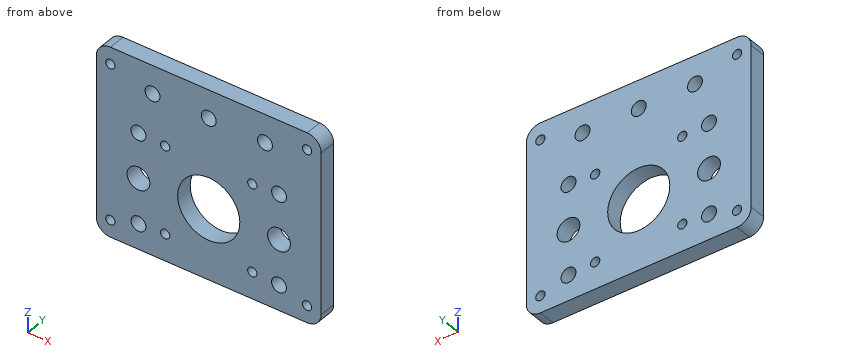
from build123d import *

# Parameters (mm, degrees)
SKETCH_1_R      = 11.05
SKETCH_1_R_2    = 1.65
SKETCH_1_R_3    = 4.05
SKETCH_1_R_4    = 2.65
EXTRUDE_1_DEPTH = 6


with BuildPart() as part:
    # 草图1 → 凸台-拉伸1 (new body)
    with BuildSketch(Plane(origin=(0, 0, 0), x_dir=(1, 0, 0), z_dir=(0, 1, 0))):
        with BuildLine():
            Line((-35, -42), (35, -42))
            ThreePointArc((35, -42), (38.535533906, -40.535533906), (40, -37))
            Line((40, -37), (40, 20))
            ThreePointArc((40, 20), (38.535533906, 23.535533906), (35, 25))
            Line((35, 25), (-35, 25))
            ThreePointArc((-35, 25), (-38.535533906, 23.535533906), (-40, 20))
            Line((-40, 20), (-40, -37))
            ThreePointArc((-40, -37), (-38.535533906, -40.535533906), (-35, -42))
        make_face()
        with Locations(Location((0, 0, 0), (0, 0, 270))):
            Circle(SKETCH_1_R, mode=Mode.SUBTRACT)
        with Locations(Location((-15.5, 15.5, 0), (0, 0, 270))):
            Circle(SKETCH_1_R_2, mode=Mode.SUBTRACT)
        with Locations(Location((15.5, 15.5, 0), (0, 0, 270))):
            Circle(SKETCH_1_R_2, mode=Mode.SUBTRACT)
        with Locations(Location((15.5, -15.5, 0), (0, 0, 270))):
            Circle(SKETCH_1_R_2, mode=Mode.SUBTRACT)
        with Locations(Location((-15.5, -15.5, 0), (0, 0, 270))):
            Circle(SKETCH_1_R_2, mode=Mode.SUBTRACT)
        with Locations(Location((-25, 0, 0), (0, 0, 270))):
            Circle(SKETCH_1_R_3, mode=Mode.SUBTRACT)
        with Locations(Location((-25, 16, 0), (0, 0, 270))):
            Circle(SKETCH_1_R_4, mode=Mode.SUBTRACT)
        with Locations(Location((-25, -16, 0), (0, 0, 90))):
            Circle(SKETCH_1_R_4, mode=Mode.SUBTRACT)
        with Locations(Location((25, 0, 0), (0, 0, 90))):
            Circle(SKETCH_1_R_3, mode=Mode.SUBTRACT)
        with Locations(Location((25, -16, 0), (0, 0, 270))):
            Circle(SKETCH_1_R_4, mode=Mode.SUBTRACT)
        with Locations(Location((25, 16, 0), (0, 0, 90))):
            Circle(SKETCH_1_R_4, mode=Mode.SUBTRACT)
        with Locations(Location((-20, -32, 0), (0, 0, 270))):
            Circle(SKETCH_1_R_4, mode=Mode.SUBTRACT)
        with Locations(Location((0, -32, 0), (0, 0, 270))):
            Circle(SKETCH_1_R_4, mode=Mode.SUBTRACT)
        with Locations(Location((20, -32, 0), (0, 0, 270))):
            Circle(SKETCH_1_R_4, mode=Mode.SUBTRACT)
        with Locations(Location((-35, 19, 0), (0, 0, 270))):
            Circle(SKETCH_1_R_2, mode=Mode.SUBTRACT)
        with Locations(Location((-35, -36, 0), (0, 0, 270))):
            Circle(SKETCH_1_R_2, mode=Mode.SUBTRACT)
        with Locations(Location((35, -36, 0), (0, 0, 90))):
            Circle(SKETCH_1_R_2, mode=Mode.SUBTRACT)
        with Locations(Location((35, 19, 0), (0, 0, 90))):
            Circle(SKETCH_1_R_2, mode=Mode.SUBTRACT)
    extrude(amount=EXTRUDE_1_DEPTH)


solid = part.part
The model under review builds one solid part; all positions refer to its coordinate system, in mm. Give positions to 0.01 mm unless a question says otherwise; leave off trailing zeros. Loops run counter-clockwise (first coordinate to the right, second up) from the corner with the lowest first, then second, coordinate; pieces in that order, holes last. Notation, with made-up numbers: (40, 42) -> (75, 42) arc R10 cw to (75, 59) -> close; hole circle Ø1 at (34.25, -29). An arc over 180 degrees is marked (long way). Answer as a JSON object with one key per item and string values. Group by question number.
Q1. Take a section at B-B (z = 32). Write out the cut boundary in (x, y), plus the area to 3 significant figures.
Q2. Take a section at A-A (x = -25). Write out the cut boundary in (y, z).
Q3. Wall thickness on line 1 along X through (y, z) = (3.2, 36); line 2 along X through (y, z) = (2.75, 0); line 3 along X through (y, z) = (1.7, 33): over which ranges is each line inside the solid? List them lowest first.
Q4. Take a section at C-C (x = 15.5). Write out the cut boundary in (y, z).
Q5. Take a section at D-D (y = 1.45). State how many separate pieces and enclosed holes the cut face has, plus the area to 3 significant figures.
Answer below:
{
 "1": {"outline": "(-40, 0) -> (-22.65, 0) -> (-22.65, 6) -> (-40, 6) -> close; (-17.35, 0) -> (-2.65, 0) -> (-2.65, 6) -> (-17.35, 6) -> close; (2.65, 0) -> (17.35, 0) -> (17.35, 6) -> (2.65, 6) -> close; (22.65, 0) -> (40, 0) -> (40, 6) -> (22.65, 6) -> close", "area": "385 mm2"},
 "2": {"outline": "(0, -25) -> (6, -25) -> (6, -18.65) -> (0, -18.65) -> close; (0, -13.35) -> (6, -13.35) -> (6, -4.05) -> (0, -4.05) -> close; (0, 4.05) -> (6, 4.05) -> (6, 13.35) -> (0, 13.35) -> close; (0, 18.65) -> (6, 18.65) -> (6, 42) -> (0, 42) -> close"},
 "3": {"line 1": "x = -40 to -36.65, -33.35 to 33.35, 36.65 to 40", "line 2": "x = -40 to -29.05, -20.95 to -11.05, 11.05 to 20.95, 29.05 to 40", "line 3": "x = -40 to -22.45, -17.55 to -2.45, 2.45 to 17.55, 22.45 to 40"},
 "4": {"outline": "(0, -25) -> (6, -25) -> (6, -17.15) -> (0, -17.15) -> close; (0, -13.85) -> (6, -13.85) -> (6, 13.85) -> (0, 13.85) -> close; (0, 17.15) -> (6, 17.15) -> (6, 42) -> (0, 42) -> close"},
 "5": {"separate pieces": "1", "enclosed holes": "18", "area": "4,630 mm2"}
}
